Autodesk Inventor part; units mm, degrees
ref_plane "Work Plane2" through (44, 0, 40.5) normal (1, 0, 0) x (0, 0, -1)
ref_plane "YZ Plane" through (0, 0, 0) normal (1, 0, 0) x (0, 1, 0)
ref_plane "XZ Plane" through (0, 0, 0) normal (0, 1, 0) x (-1, 0, 0)
sketch "Sketch1" plane through (0, 0, 0) normal (0, 0, 1) x (1, 0, 0)
  line L0 (0, 0) -> (44, 0)
  line L1 (44, 0) -> (44, 9.6635)
  line L2 (44, 9.6635) -> (0, 9.6635)
  line L3 (0, 9.6635) -> (0, 0)
  circle A0 centre (5, 4.8317) radius 3
  circle A1 centre (39, 4.8317) radius 3
  dimension "d0" = 6
  dimension "d1" = 6
  dimension "d2" = 34
  dimension "d3" = 44
  dimension "d4" = 5
extrude "Extrusion1" add sketch "Sketch1" along normal blind 42.5
sketch "Sketch2" plane through (0, 9.6635, 0) normal (0, 1, 0) x (1, 0, 0)
  line L0 (44, 0) -> (0, 0)
  line L1 (0, 0) -> (0, -42.5)
  line L2 (8, -42.5) -> (42, -42.5)
  point P0 (11, -32.5)
  point P1 (0, -40.5)
  dimension "d17" = 10
  dimension "d18" = 11
hole "Hole1" at (11, 9.6635, 32.5) direction (0, -1, 0) diameter 4 depth 10 tip angle 118
sketch "Sketch3" plane through (0, 9.6635, 0) normal (0, 1, 0) x (1, 0, 0)
  line L0 (8, -42.5) -> (42, -42.5)
  line L1 (44, 0) -> (44, -42.5)
  point P0 (0, 0)
  point P1 (34, -32.5)
  point P2 (44, -40.5)
  dimension "d19" = 10
  dimension "d20" = 10
hole "Hole2" at (34, 9.6635, 32.5) direction (0, -1, 0) diameter 4 depth 10 tip angle 118
sketch "Sketch4" plane through (0, 0, 0) normal (0, 0, -1) x (-1, 0, 0)
  line L0 (0, -7.5) -> (-44, -7.5)
  line L1 (-44, -7.5) -> (-44, 0)
  line L2 (-44, 0) -> (0, 0)
  line L3 (0, 0) -> (0, -7.5)
  line L4 (-44, 9.6635) -> (0, 9.6635)
  line L5 (0, 9.6635) -> (0, 37.1635)
  line L6 (0, 37.1635) -> (-44, 37.1635)
  line L7 (-44, 37.1635) -> (-44, 9.6635)
  circle A0 centre (-39, 4.8317) radius 3
  circle A1 centre (-5, 4.8317) radius 3
  line L8 (0, 0) -> (-44, 0)
  line L9 (0, 9.6635) -> (0, 0)
  line L10 (-44, 9.6635) -> (0, 9.6635)
  line L11 (-44, 0) -> (-44, 9.6635)
  dimension "d28" = 7.5
  dimension "d29" = 27.5
extrude "Extrusion2" add sketch "Sketch4" along normal blind 20
sketch "Sketch5" plane through (0, 0, -20) normal (0, 0, -1) x (-1, 0, 0)
  arc A0 (-8, 4.8317) -> (-8, 4.8317) centre (-5, 4.8317) ccw
  circle A1 centre (-5, 4.8317) radius 3
  circle A2 centre (-39, 4.8317) radius 3
  circle A3 centre (-39, 4.8317) radius 3
  point P0 (0, 0)
extrude "Extrusion3" add sketch "Sketch5" against normal blind 20
ref_plane "Work Plane2" through (44, 0, 40.5) normal (1, 0, 0) x (0, 0, -1)
sketch "Sketch6" plane through (44, 0, 40.5) normal (1, 0, 0) x (0, 0, -1)
  line L0 (55.5, 37.1635) -> (45.5, 37.1635)
  line L1 (45.5, 37.1635) -> (45.5, 25.1635)
  line L2 (45.5, 25.1635) -> (55.5, 25.1635)
  line L3 (55.5, 25.1635) -> (55.5, 37.1635)
  line L4 (60.5, 37.1635) -> (60.5, -7.5)
  line L5 (40.5, -7.5) -> (60.5, -7.5)
  line L6 (55.5, -7.5) -> (45.5, -7.5)
  line L7 (45.5, -7.5) -> (45.5, 4.5)
  line L8 (45.5, 4.5) -> (55.5, 4.5)
  line L9 (55.5, 4.5) -> (55.5, -7.5)
  line L10 (40.5, 37.1635) -> (60.5, 37.1635)
  point P0 (40.5, 0)
  dimension "d34" = 10
  dimension "d35" = 5
  dimension "d36" = 12
  dimension "d37" = 12
  dimension "d55" = 0
extrude "Extrusion4" cut sketch "Sketch6" against normal through all
sketch "Sketch7" plane through (0, 0, -20) normal (0, 0, -1) x (-1, 0, 0)
  line L0 (0, 0) -> (-44, 0)
  line L1 (0, 37.1635) -> (-44, 37.1635)
  line L2 (-44, -7.5) -> (0, -7.5)
  line L3 (0, -7.5) -> (0, 37.1635)
  line L4 (-44, 37.1635) -> (-44, -7.5)
  point P0 (-37, -3.5)
  point P1 (-7, 33.1635)
  point P2 (-37, 33.1635)
  point P3 (-7, -3.5)
  dimension "d40" = 4
  dimension "d41" = 4
  dimension "d42" = 4
  dimension "d43" = 4
  dimension "d44" = 7
  dimension "d45" = 7
  dimension "d46" = 7
  dimension "d47" = 7
hole "Hole3" at (37, -3.5, -20) at (7, 33.1635, -20) at (37, 33.1635, -20) at (7, -3.5, -20) direction (0, 0, 1) diameter 4 depth 16 tip angle 118 counterbore diameter 5 counterbore depth 6
sketch "Sketch8" plane through (0, 0, 0) normal (0, 0, 1) x (1, 0, 0)
  line L0 (44, 25.1635) -> (0, 25.1635)
  line L1 (0, 9.6635) -> (5, 9.6635)
  line L2 (5, 9.6635) -> (5, 25.1635)
  line L3 (5, 25.1635) -> (0, 25.1635)
  line L4 (0, 25.1635) -> (0, 9.6635)
  point P0 (0, 0)
  dimension "d56" = 5
extrude "Extrusion5" add sketch "Sketch8" along normal blind 15.5
chamfer "Chamfer1" distance 15.5 angle 45 1 edges at (2.5, 25.1635, 15.5)
sketch "Sketch9" plane through (5, 9.6635, 0) normal (1, 0, 0) x (0, 0, -1)
  line L0 (-15.5, 0) -> (0, 15.5)
  line L1 (0, 0) -> (-15.5, 0)
  line L2 (0, 15.5) -> (0, 0)
  point P0 (0, -9.6635)
extrude "Extrusion6" add sketch "Sketch9" along normal up to surface (39 mm away)
sketch "Sketch11" plane through (44, 0, 42.5) normal (1, 0, 0) x (0, 0, -1)
  line L0 (42.5, 25.1635) -> (33.1498, 9.6635)
  line L1 (33.1498, 9.6635) -> (27, 9.6635)
  line L2 (27, 9.6635) -> (42.5, 25.1635)
  line L3 (42.5, 25.1635) -> (27, 9.6635)
  point P0 (42.5, 0)
extrude "Extrusion7" cut sketch "Sketch11" against normal through all
properties part number "X smooth mount"
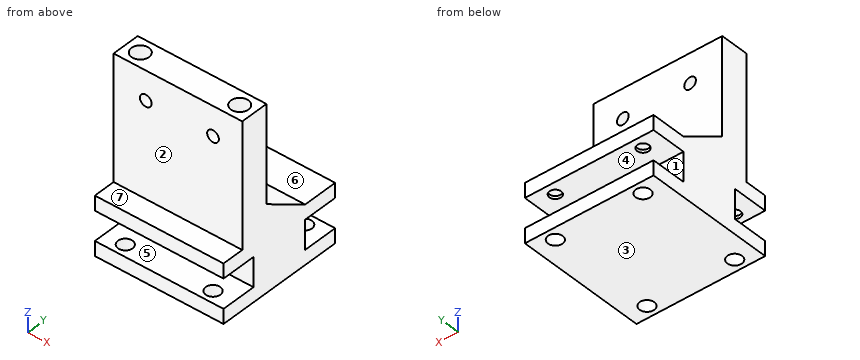
Design review of the part built by this model. Coordinates are the model's own, in mm. Face numbers are marked on the shaded views. A direction names the side the tool comes from. Give positions to 0.01 mm unless a question says otherwise; leave off trailing zeros. Write each loop counter-clockwise with the first axis right and the second up, starting at its lowest first coordinate (ties: lowest second). Pieces come first, ordered by that corner, then holes. Notation, with made-up numbers: (-34.75, -5) - (20.25, -5) arc R26 cw to (20.25, 24) - close; hole circle Ø5 at (-22, -39). An arc over 180 degrees is marked (long way). Return JSON: item names as keys, results as strings. Group by question number.
(1) We need section A-A, the plane z = 31.5. Give the boundary of the cut face in (x, y), then the cut area to 3 significant figures.
(2) We need section D-D, the plane z = 25. Give the boundary of the cut face in (x, y), then the cut area to 3 significant figures.
(3) Mouldability with a two-part tool opening along Z and no side actions: class the marked faces 1, 2 and 3 as +Z half, -Z half, draft (parallel to the pull), parting line (faces both ways), or undercut.
(4) Machinability: for the marked faces 4, 5, 6 and 7, which of the approach directions +Z, -Z, +X, -X, +Y, -Y give a long, thin tool a straight path to every point of the face, cutting with its end or side? Answer none if there is none.
(5) We need section C-C, the plane x = 21. Give the boundary of the cut face in (y, z).
(6) To check wall thickness, follow probe 1 along Y at (x, z) = (37, -17.5); probe 2 along X at (y, z) = (1.5, 32.5); probe 3 along Y at (x, z) = (7, -4.45). State the ranges of each line that lie inside material, in increasing order.
(7) We need section B-B, the plane y = 6.5. Give the boundary of the cut face in (x, z).
(8) Insertion check: pin 1 (3 mm diameter, centred on x = 24.5, z = -8, fed in from -Y); pin 2 (1 mm diameter, centred on x = 39, y = 24, fed in from +Z); pin 3 (4.5 mm diameter, centred on x = 37, y = 33.16, fed in from -Z); pin 4 (3.5 mm diameter, centred on x = 34, z = 32.5, fed in from +Y). Each pin has a flat end and moves straight along its axis. Give the tip position at first contact, or say it passes through.
Reported:
{
 "1": {"outline": "(0, 0) - (9.27, 0) - (9.27, 9.66) - (0, 9.66) - close; (12.73, 0) - (32.27, 0) - (32.27, 9.66) - (12.73, 9.66) - close; (35.73, 0) - (44, 0) - (44, 9.66) - (35.73, 9.66) - close; hole circle Ø6 at (5, 4.83); hole circle Ø6 at (39, 4.83)", "area": "302 mm2"},
 "2": {"outline": "(0, 0) - (44, 0) - (44, 9.66) - (0, 9.66) - close; hole circle Ø6 at (5, 4.83); hole circle Ø6 at (39, 4.83)", "area": "369 mm2"},
 "3": {"face 1": "undercut", "face 2": "draft", "face 3": "-Z half"},
 "4": {"face 4": "+X, -X, +Y", "face 5": "+X, -X, -Y", "face 6": "+Z, +X, -X, +Y", "face 7": "+Z, +X, -X, -Y"},
 "5": {"outline": "(-7.5, -20) - (37.16, -20) - (37.16, -15) - (25.16, -15) - (25.16, -5) - (37.16, -5) - (37.16, 0) - (25.16, 0) - (9.66, 9.35) - (9.66, 42.5) - (0, 42.5) - (0, 0) - (-7.5, 0) - (-7.5, -5) - (4.5, -5) - (4.5, -15) - (-7.5, -15) - close"},
 "6": {"probe 1": "y = -7.5 to -6, -1 to 30.66, 35.66 to 37.16", "probe 2": "x = 0 to 9, 13 to 32, 36 to 44", "probe 3": "y = -7.5 to -5.5, -1.5 to 31.16, 35.16 to 37.16"},
 "7": {"outline": "(0, -20) - (44, -20) - (44, 42.5) - (41.49, 42.5) - (41.49, 0) - (36.51, 0) - (36.51, 42.5) - (7.49, 42.5) - (7.49, 0) - (2.51, 0) - (2.51, 42.5) - (0, 42.5) - close; hole circle Ø4 at (11, 32.5); hole circle Ø4 at (34, 32.5)"},
 "8": {"pin 1": "stops at y = 4.5", "pin 2": "stops at z = 1", "pin 3": "stops at z = -5", "pin 4": "passes through"}
}
